from build123d import *

# Parameters (mm, degrees)
F2_DEPTH = 914.4
F4_DEPTH = 50.801
F6_DEPTH = 50.801
F7_R     = 3.175


# Not quite as in the source:
# - a variable given as a bare number and used for a length is read in inches; the dataset says mm whatever the document's units were


with BuildPart() as f2:
    # F0 (on Front) → F2 (new body)
    with BuildSketch(Plane.XZ):
        Polygon((-38.1, 22.225), (-38.1, -22.225), (-38.1, -25.4), (-34.925, -25.4), (34.925, -25.4), (38.1, -25.4), (38.1, -22.225), (38.1, 22.225), (38.1, 25.4), (34.925, 25.4), (-34.925, 25.4), (-38.1, 25.4), align=None)
        with BuildLine():
            ThreePointArc((31.75, 22.225), (33.9950640303, 21.2950640303), (34.925, 19.05))
            Line((34.925, 19.05), (34.925, -19.05))
            ThreePointArc((34.925, -19.05), (33.9950640303, -21.2950640303), (31.75, -22.225))
            Line((31.75, -22.225), (-31.75, -22.225))
            ThreePointArc((-31.75, -22.225), (-33.9950640303, -21.2950640303), (-34.925, -19.05))
            Line((-34.925, -19.05), (-34.925, 19.05))
            ThreePointArc((-34.925, 19.05), (-33.9950640303, 21.2950640303), (-31.75, 22.225))
            Line((-31.75, 22.225), (31.75, 22.225))
        make_face(mode=Mode.SUBTRACT)
    extrude(amount=F2_DEPTH)

    # F3 (on face) → F4 (cut, through all)
    with BuildSketch(Plane.XY.offset(25.4)):
        Polygon((38.1, 0), (-38.1, 0), (-38.1, -76.2), align=None)
    extrude(amount=-F4_DEPTH, mode=Mode.SUBTRACT)

    # F5 (on face) → F6 (cut, through all)
    with BuildSketch(Plane.XY.offset(25.4)):
        Polygon((-38.1, -914.4), (38.1, -914.4), (-38.1, -838.2), align=None)
    extrude(amount=-F6_DEPTH, mode=Mode.SUBTRACT)

    # F7
    f7_edges = [f2.edges().sort_by_distance(p)[0] for p in [
        (-38.1, -457.2, 25.4),
        (-38.1, -457.2, -25.4),
        (38.1, -457.2, 25.4),
        (38.1, -457.2, -25.4),
    ]]
    fillet(f7_edges, radius=F7_R)


solid = f2.part
Verification items for the finished model (mm, model axes). A direction names the side the tool comes from. Coordinates: 2 decimals unless noted, no trailing zeros. Order: outer loops, then holes, each group sorted by start corner. A loop starts at its lowest first (then second) coordinate and runs counter-clockwise, first axis right, second up. Notation, with made-up numbers: M -2,54.25 L 28,54.25 A21 cw 28,75.25 Z; hole C 50,50.25 d9. An arc over 180 degrees is marked long. One line per item, written item: value. Start each with the question number.
Item 1: Mould release check, pull along Z, two halves, no side actions. Record for faces 1 (the flat face through (0, -451, 25.4)), 2 (the flat face through (-38.1, -452, 0)), 3 (the flat face through (-34.925, -452, 0)), 4 (the flat face through (0, -451, -25.4)): released by +Z, released by -Z, zero draft, split by the parting line, or undercut.
Item 2: Scan lines: probe 1 along Z at (x, y) = (-6, -126) (3 decimals); probe 2 along X at (y, z) = (-272, 20); probe 3 along X at (y, z) = (-396, -3) (3 decimals). Record each from-to range of solid material in increasing order.
Item 3: Access from +Z, -Z, +X, -X, +Y, -Y to the whole of each face (thin tool, end or side, straight path). Record for faces 5 (the flat face through (34.925, -451, 0)), 6 (the flat face through (38.1, -451, 0)).
Item 4: Sectioned sample at A-A (x = 0). Enter the section's corners in (y, z) (3 decimals).
Item 5: Sectioned sample at B-B (z = 8). Enter the section's corners in (x, y) (3 decimals).
Item 6: Sectioned sample at C-C (y = -284). Enter the section's corners in (x, z) (3 decimals), then the cut area to 3 significant figures.
Conclusion:
1. face 1: released by +Z
1. face 2: zero draft
1. face 3: undercut
1. face 4: released by -Z
2. probe 1: z = -25.4 to -22.225, 22.225 to 25.4
2. probe 2: x = -38.1 to -34.78, 34.78 to 38.1
2. probe 3: x = -38.1 to -34.925, 34.925 to 38.1
3. face 5: +Y, -Y
3. face 6: +Z, -Z, +X, +Y, -Y
4. outline: M -876.3,-25.4 L -38.1,-25.4 L -38.1,-22.225 L -876.3,-22.225 Z; M -876.3,22.225 L -38.1,22.225 L -38.1,25.4 L -876.3,25.4 Z
5. outline: M -38.1,-838.2 L -34.925,-841.375 L -34.925,-73.025 L -38.1,-76.2 Z; M 34.925,-911.225 L 38.1,-914.4 L 38.1,0 L 34.925,-3.175 Z
6. outline: M -38.1,-22.225 A3.175 ccw -34.925,-25.4 L 34.925,-25.4 A3.175 ccw 38.1,-22.225 L 38.1,22.225 A3.175 ccw 34.925,25.4 L -34.925,25.4 A3.175 ccw -38.1,22.225 Z; hole M -34.925,-19.05 A3.175 ccw -31.75,-22.225 L 31.75,-22.225 A3.175 ccw 34.925,-19.05 L 34.925,19.05 A3.175 ccw 31.75,22.225 L -31.75,22.225 A3.175 ccw -34.925,19.05 Z
6. area: 766 mm^2
